Autodesk Inventor part; units mm, degrees
ref_plane "Work Plane1" through (-2.5, 0, -17) normal (-1, 0, 0) x (0, 0, 1)
ref_plane "YZ Plane" through (0, 0, 0) normal (1, 0, 0) x (0, 1, 0)
ref_plane "XZ Plane" through (0, 0, 0) normal (0, 1, 0) x (-1, 0, 0)
sketch "Sketch1" plane through (0, 0, 0) normal (0, 1, 0) x (-1, 0, 0)
  line L0 (0, 0) -> (5, 0)
  line L1 (5, 0) -> (5, -17)
  line L2 (5, -17) -> (0, -17)
  line L3 (0, -17) -> (0, 0)
  dimension "d0" = 5
  dimension "d1" = 17
extrude "Extrusion1" add sketch "Sketch1" along normal blind 40
sketch "Sketch2" plane through (-5, 0, -17) normal (-1, 0, 0) x (0, 0, 1)
  line L0 (17, 0) -> (17, 40)
  line L1 (17, 20) -> (-0.1378, 20)
  circle A0 centre (7, 20) radius 2
  line L2 (0, 0) -> (17, 0)
  line L3 (6.5, -6.3182) -> (6.5, 42.5723) construction
  line L4 (0, 0) -> (0, 40)
  circle A1 centre (6.5, 8.5109) radius 0.5
  circle A2 centre (7, 31.5) radius 0.5
  dimension "d4" = 4
  dimension "d7" = 6.5
  dimension "d9" = 11.5
  dimension "d10" = 1
  dimension "d11" = 1
  dimension "d12" = 0.5
  dimension "d13" = 11.5
  dimension "d105" = 7
extrude "Extrusion2" cut sketch "Sketch2" against normal through all contours A0 L1 | L1 A0 | A1 | A2
hole "Hole1" at (-5, 8.5109, -10.5) direction (1, 0, 0) diameter 2.4 end through all
hole "Hole2" at (-5, 31.5, -10) direction (1, 0, 0) diameter 2.4 end through all
sketch "Sketch3" plane through (-5, 0, -17) normal (-1, 0, 0) x (0, 0, 1)
  circle A0 centre (7, 20) radius 2
  circle A1 centre (7, 20) radius 5 construction
  line L0 (7, 20) -> (16.0941, 20)
  circle A2 centre (12, 20) radius 0.5
  circle A3 centre (9.5, 24.3301) radius 0.5
  circle A4 centre (4.5, 24.3301) radius 0.5
  circle A5 centre (2, 20) radius 0.5
  circle A6 centre (4.5, 15.6699) radius 0.5
  circle A7 centre (9.5, 15.6699) radius 0.5
  point P0 (17, 0)
  dimension "d32" = 10
  dimension "d33" = 1
  dimension "d36" = 360
extrude "Extrusion3" cut sketch "Sketch3" against normal through all contours A2 L0 | L0 A2 | A3 | A4 | A5 | A6 | A7
hole "Hole3" at (-5, 20, -5) direction (1, 0, 0) diameter 1.8 end through all countersink diameter 3.6 countersink angle 90
hole "Hole4" at (-5, 15.6699, -7.5) direction (1, 0, 0) diameter 1.8 end through all countersink diameter 3.6 countersink angle 90
hole "Hole5" at (-5, 15.6699, -12.5) direction (1, 0, 0) diameter 1.8 end through all countersink diameter 3.6 countersink angle 90
hole "Hole6" at (-5, 20, -15) direction (1, 0, 0) diameter 1.8 end through all countersink diameter 3.6 countersink angle 90
hole "Hole7" at (-5, 24.3301, -12.5) direction (1, 0, 0) diameter 1.8 end through all countersink diameter 3.6 countersink angle 90
hole "Hole8" at (-5, 24.3301, -7.5) direction (1, 0, 0) diameter 1.8 end through all countersink diameter 3.6 countersink angle 90
ref_plane "Work Plane1" through (-2.5, 0, -17) normal (-1, 0, 0) x (0, 0, 1)
mirror "Mirror1" about plane through (-2.5, 0, -17) normal (-1, 0, 0) of "Hole6", "Hole5", "Hole4", "Hole3", "Hole8", "Hole7"
sketch "Sketch6" plane through (-5, 0, -17) normal (-1, 0, 0) x (0, 0, 1)
  circle A0 centre (7, 20) radius 2
  circle A1 centre (7, 20) radius 9
  point P0 (17, 0)
  dimension "d102" = 18
extrude "Extrusion6" cut sketch "Sketch6" against normal blind 2.5
properties part number "mounting"
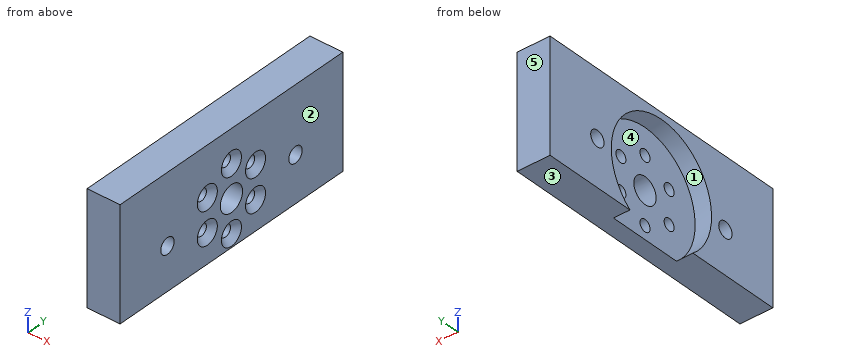
Check sheet for the modelled part. Datum: model origin and axes. Units: mm. Face numbers are marked on the shaded views. A direction names the side the tool comes from. Coordinates: 2 decimals unless noted, no trailing zeros. Write each loop counter-clockwise with the first axis right and the second up, starting at its lowest first coordinate (ties: lowest second). Pieces come first, ordered by that corner, then holes. Notation, with made-up numbers: M 57,-3 L 101,-3 A25 cw 101,11 Z; hole C -30.5,79 d3. An arc over 180 degrees is marked long. Write item = value, one per line. Start each with the question number.
1. Tool access check on the marked faces 1 and 2. Record the directions out of +Z, -Z, +X, -X, +Y, -Y that give a thin tool (end or side, any length) a straight path to the whole face; none if there is none.
2. Sectioned sample at A-A (y = 20). Record the cut outline in (x, z), then the cut area to 3 significant figures.
3. Thickness scan on probe 1 along Y at (x, z) = (-1.45, -10); probe 2 along Y at (x, z) = (-2, -5); probe 3 along Y at (x, z) = (-2.1, -11.75). Record the ranges inside material, lowest first.
4. Sectioned sample at C-C (y = 31.5). Record the cut outline in (x, z), then the cut area to 3 significant figures.
5. Sectioned sample at B-B (z = -12.5). Record the cut outline in (x, y).
6. Go/stop test with flat-tipped pins: pin 1 (2.5 mm diameter, centred on y = 15.67, z = -12.5, fed in from +X); pin 2 (2 mm diameter, centred on x = -3.5, y = 4, fed in from +Z); pin 3 (3 mm diameter, centred on y = 18, z = -12.5, fed in from -X); pin 4 (3 mm diameter, centred on y = 20, z = -5, fed in from +X). Record where each tip stops, or that it passes through.
7. Mould release check, pull along Z, two halves, no side actions. Record for the marked faces 3, 4 and 5: pulls with the +Z half, pulls with the -Z half, needs draft (parallel to the pull), parting line crosses it, or undercut.
8. Sectioned sample at D-D (x = -1.7). State how many separate pieces and enclosed holes the cut face has, then the cut area to 3 significant figures.
The answers:
q1.face_1 = -X
q1.face_2 = +Z, -Z, +X, +Y, -Y
q2.outline = M -5,-1 L -2.5,-1 L -2.5,-4.1 L -0.9,-4.1 L 0,-3.2 L 0,0 L -5,0 Z; M -2.5,-17 L 0,-17 L 0,-16.8 L -0.9,-15.9 L -2.5,-15.9 Z; M -2.5,-14.1 L -0.9,-14.1 L 0,-13.2 L 0,-12 L -2.5,-12 Z; M -2.5,-8 L 0,-8 L 0,-6.8 L -0.9,-5.9 L -2.5,-5.9 Z
q2.area = 24.4 mm²
q3.probe_1 = 0 to 7.42, 9.6 to 18, 22 to 30.3, 32.7 to 40
q3.probe_2 = 0 to 19.1, 20.9 to 40
q3.probe_3 = 0 to 15.17, 16.17 to 19.03, 20.97 to 23.83, 24.83 to 40
q4.outline = M -5,-17 L 0,-17 L 0,-11.2 L -5,-11.2 Z; M -5,-8.8 L 0,-8.8 L 0,0 L -5,0 Z
q4.area = 73.0 mm²
q5.outline = M -5,0 L 0,0 L 0,13.87 L -0.9,14.77 L -2.5,14.77 L -2.5,11.35 L -5,11.35 Z; M -5,28.65 L -2.5,28.65 L -2.5,25.23 L -0.9,25.23 L 0,26.13 L 0,40 L -5,40 Z; M -2.5,16.57 L -0.9,16.57 L 0,17.47 L 0,22.53 L -0.9,23.43 L -2.5,23.43 Z
q6.pin_1 = -0.55
q6.pin_2 = 0
q6.pin_3 = -2.5
q6.pin_4 = -0.3
q7.face_3 = pulls with the -Z half
q7.face_4 = undercut
q7.face_5 = needs draft
q8.separate_pieces = 1
q8.enclosed_holes = 9
q8.area = 643 mm²
